```python
from build123d import *

# Parameters (mm, degrees)
SKETCH1_W           = 2
SKETCH1_H           = 50
SKETCH1_H_2         = 15
BOSS_EXTRUDE1_DEPTH = 10
SKETCH2_W           = 8.2
SKETCH2_H           = 3
BOSS_EXTRUDE2_DEPTH = 10
SKETCH3_R           = 3.175
CUT_EXTRUDE1_DEPTH  = 30
CUT_EXTRUDE2_DEPTH  = 30
BOSS_EXTRUDE3_DEPTH = 10
SKETCH6_W           = 4.7
SKETCH6_H           = 10
BOSS_EXTRUDE4_DEPTH = 10
SKETCH7_R           = 1.91
CUT_EXTRUDE3_DEPTH  = 10
CUT_EXTRUDE4_DEPTH  = 10
FILLET1_R           = 0.2


with BuildPart() as part:
    # Sketch1 → Boss-Extrude1 (new body)
    with BuildSketch(Plane.XY):
        with Locations((-1, -25)):
            Rectangle(SKETCH1_W, SKETCH1_H)
        Polygon((-2, 0), (0, 0), (6.3, 0), (8.3, 0), (8.3, 2), (-2, 2), align=None)
        with Locations((7.3, -7.5)):
            Rectangle(SKETCH1_W, SKETCH1_H_2)
    extrude(amount=BOSS_EXTRUDE1_DEPTH)

    # Sketch2 → Boss-Extrude2 (add)
    with BuildSketch(Plane.XY.offset(10)):
        with Locations((-6.1, -48.5)):
            Rectangle(SKETCH2_W, SKETCH2_H)
        with Locations((-6.1, -21.5)):
            Rectangle(SKETCH2_W, SKETCH2_H)
    extrude(amount=-BOSS_EXTRUDE2_DEPTH)

    # Sketch3 → Cut-Extrude1 (cut)
    with BuildSketch(Plane(origin=(0, -20, 0), x_dir=(1, 0, 0), z_dir=(0, 1, 0))):
        with Locations((-5.175, -5)):
            Circle(SKETCH3_R)
    extrude(amount=-CUT_EXTRUDE1_DEPTH, mode=Mode.SUBTRACT)

    # Sketch4 → Cut-Extrude2 (cut)
    with BuildSketch(Plane(origin=(0, -20, 0), x_dir=(1, 0, 0), z_dir=(0, 1, 0))):
        with BuildLine():
            Line((-5.67562461, 0), (-10.2, 0))
            Line((-10.2, 0), (-10.2, -5))
            ThreePointArc((-10.2, -5), (-8.901007492, -1.62842868), (-5.67562461, 0))
        make_face()
        with BuildLine():
            ThreePointArc((-5.67562461, -10), (-8.901007492, -8.37157132), (-10.2, -5))
            Line((-10.2, -5), (-10.2, -10))
            Line((-10.2, -10), (-5.67562461, -10))
        make_face()
    extrude(amount=-CUT_EXTRUDE2_DEPTH, mode=Mode.SUBTRACT)

    # Sketch5 → Boss-Extrude3 (add)
    with BuildSketch(Plane.XY.offset(10)):
        with BuildLine():
            Line((-2, 2), (0, 2))
            ThreePointArc((0, 2), (3.15, 5.15), (6.3, 2))
            Line((6.3, 2), (8.3, 2))
            ThreePointArc((8.3, 2), (3.15, 7.15), (-2, 2))
        make_face()
    extrude(amount=-BOSS_EXTRUDE3_DEPTH)

    # Sketch6 → Boss-Extrude4 (add)
    with BuildSketch(Plane.XY.offset(10)):
        with Locations((10.65, -5)):
            Rectangle(SKETCH6_W, SKETCH6_H)
    extrude(amount=-BOSS_EXTRUDE4_DEPTH)

    # Sketch7 → Cut-Extrude3 (cut)
    with BuildSketch(Plane(origin=(0, 0, 0), x_dir=(1, 0, 0), z_dir=(0, 1, 0))):
        with Locations((10.21, -5)):
            Circle(SKETCH7_R)
    extrude(amount=-CUT_EXTRUDE3_DEPTH, mode=Mode.SUBTRACT)

    # Sketch8 → Cut-Extrude4 (cut)
    with BuildSketch(Plane(origin=(0, 0, 0), x_dir=(1, 0, 0), z_dir=(0, 1, 0))):
        with BuildLine():
            Line((13, -6.6), (13, -10))
            Line((13, -10), (8.3, -10))
            Line((8.3, -10), (8.3, -5))
            ThreePointArc((8.3, -5), (9.30012633, -6.679354014), (11.253120319, -6.6))
            Line((11.253120319, -6.6), (13, -6.6))
        make_face()
    extrude(amount=-CUT_EXTRUDE4_DEPTH, mode=Mode.SUBTRACT)

    # Fillet1
    fillet1_edges = [part.edges().sort_by_distance(p)[0] for p in [
        (11.253120319, -5, 6.6),
    ]]
    fillet(fillet1_edges, radius=FILLET1_R)


solid = part.part
```
Here's how the part is built. I have some questions about the finished solid (model axes, mm). A direction names the side the tool comes from. Round coordinates to 2 decimals unless told otherwise and drop trailing zeros. Write each loop counter-clockwise with the first axis right and the second up, starting at its lowest first coordinate (ties: lowest second). Pieces come first, ordered by that corner, then holes.
Q1. Will these pins go through, and if not, where does the flat tip stop? P1, Ø2.5, axis at x = 10.21, z = 5, coming from the +Y side; P2, Ø0.6, axis at x = 7.5, z = 7.5, coming from the -Y side; P3, Ø0.6, axis at x = 12.5, y = -6, coming from the +Z side; P4, Ø1, axis at x = 1.5, z = 6.5, coming from the +Y side.
Q2. If we section it at B-B on x = 3.15: Write out the boundary of the cut face in (y, z).
Q3. Which directions (+Z, -Z, +X, -X, +Y, -Y) give clear straight access to the entire face, cutting with the end or side of a thin tool? Please do faces 1 (the flat face through (11, -10, 3)), 2 (the flat face through (3, 2, 5)), 3 (the flat face through (11, 0, 3)), 4 (the flat face through (-9, -23, 5)).
Q4. Please list where these lines run through material, in increasing order: probe 1 along X at (y, z) = (-5.25, 5); probe 2 along X at (y, z) = (-49.1, 5); probe 3 along X at (y, z) = (-2, 7.5).
Q5. If we section it at A-A on z = 5.5: Give the number of separate pieces and of enclosed holes in the cut face, plus the area to 3 significant figures.
Q6. If we section it at C-C on y = -7: Write out the boundary of the cut face in (x, z).
Q7. If we mould it in two halves opening along Z, with no side actions, what happens to faces 5 (the flat face through (-9, -20, 5)), 6 (the cylindrical face through (-3.71, -48.479, 7.817)), 7 (the flat face through (12, -5, 6.6))? For each: +Z half, -Z half, draft (parallel to the pull), parting line (faces both ways), or undercut.
Q8. If we section it at D-D on x = -7.75: Write out the boundary of the cut face in (y, z), plus the area to 3 significant figures.
Answer below:
1. P1: passes through
1. P2: stops at y = -15
1. P3: stops at z = 6.6
1. P4: stops at y = 7.02
2. outline: (0, 0) - (2, 0) - (2, 10) - (0, 10) - close; (5.15, 0) - (7.15, 0) - (7.15, 10) - (5.15, 10) - close
3. face 1: +Z, -Z, +X, -Y
3. face 2: +Z, -Z
3. face 3: +Z, -Z, +X, +Y
3. face 4: +Z, -Z, -X
4. probe 1: x = -2 to 0, 6.3 to 8.3, 12.12 to 13
4. probe 2: x = -10.2 to -8.35, -2 to 0
4. probe 3: x = -2 to 0, 6.3 to 8.3
5. separate pieces: 4
5. enclosed holes: 1
5. area: 198 mm2
6. outline: (-2, 0) - (0, 0) - (0, 10) - (-2, 10) - close; (6.3, 0) - (13, 0) - (13, 6.6) - (11.79, 6.6) arc R0.2 ccw to (11.64, 6.27) arc R1.91 cw (long way) to (8.3, 5) - (8.3, 10) - (6.3, 10) - close
7. face 5: draft
7. face 6: undercut
7. face 7: +Z half
8. outline: (-50, 0.68) - (-47, 0.68) - (-47, 3.14) - (-50, 3.14) - close; (-50, 6.86) - (-47, 6.86) - (-47, 9.32) - (-50, 9.32) - close; (-23, 0.68) - (-20, 0.68) - (-20, 3.14) - (-23, 3.14) - close; (-23, 6.86) - (-20, 6.86) - (-20, 9.32) - (-23, 9.32) - close
8. area: 29.5 mm2
